Geometry: final body of the model. Coordinates: model frame, mm. A direction names the side the tool comes from. Coordinates: 2 decimals unless noted, no trailing zeros. Loops run counter-clockwise (first coordinate to the right, second up) from the corner with the lowest first, then second, coordinate; pieces in that order, holes last. Notation, with made-up numbers: (86.25, -34.5) - (140.25, -34.5) arc R20 ccw to (140.25, -16.5) - close; hole circle Ø5 at (74.5, 34). An arc over 180 degrees is marked (long way). Return JSON: item names as keys, results as strings.
Autodesk Inventor part; units mm, degrees
ref_plane "YZ Plane" through (0, 0, 0) normal (1, 0, 0) x (0, 1, 0)
ref_plane "XZ Plane" through (0, 0, 0) normal (0, 1, 0) x (-1, 0, 0)
ref_plane "XY Plane" through (0, 0, 0) normal (0, 0, 1) x (1, 0, 0)
sketch "Sketch1" plane through (0, 0, 0) normal (0, 1, 0) x (-1, 0, 0)
  line L0 (0, 0) -> (85.48, 0)
  line L1 (85.48, 0) -> (85.48, -127.76)
  line L2 (85.48, -127.76) -> (0, -127.76)
  line L3 (0, -127.76) -> (0, 0)
  line L4 (85.48, 0) -> (67.5195, -17.9605)
  line L5 (85.48, 0) -> (110.88, 0) construction
  line L6 (0, 0) -> (17.9605, -17.9605)
  line L7 (85.48, -127.76) -> (67.5195, -109.7995)
  line L8 (85.48, -127.76) -> (110.88, -127.76) construction
  line L9 (0, -127.76) -> (17.9605, -109.7995)
  line L10 (0, -127.76) -> (25.4, -127.76) construction
  dimension "d0" = 85.48
  dimension "d1" = 127.76
  dimension "d2" = 25.4
  dimension "d3" = 135
  dimension "d4" = 25.4
  dimension "d5" = 25.4
  dimension "d6" = 135
  dimension "d7" = 25.4
  dimension "d8" = 45
extrude "Extrusion1" add sketch "Sketch1" along normal blind 47.7
sketch "Sketch2" plane through (0, 0, 0) normal (0, -1, 0) x (1, 0, 0)
  line L0 (-85.48, 0) -> (0, 0)
  line L1 (0, 0) -> (-17.9605, -17.9605)
  line L2 (0, 0) -> (25.4, 0) construction
  line L3 (0, 0) -> (0, -127.76)
  line L4 (0, -127.76) -> (-17.9605, -109.7995)
  line L5 (0, -127.76) -> (25.4, -127.76) construction
  line L6 (-85.48, -127.76) -> (-85.48, 0)
  line L7 (-85.48, 0) -> (-67.5195, -17.9605)
  line L8 (-85.48, 0) -> (-60.08, 0) construction
  line L9 (0, -127.76) -> (-85.48, -127.76)
  line L10 (-85.48, -127.76) -> (-67.5195, -109.7995)
  line L11 (-85.48, -127.76) -> (-60.08, -127.76) construction
  dimension "d11" = 25.4
  dimension "d12" = 135
  dimension "d13" = 25.4
  dimension "d14" = 135
  dimension "d15" = 25.4
  dimension "d16" = 45
  dimension "d17" = 25.4
  dimension "d18" = 45
hole "Hole1" at (-17.9605, 0, -17.9605) at (-67.5195, 0, -17.9605) at (-67.5195, 0, -109.7995) at (-17.9605, 0, -109.7995) direction (0, 1, 0) diameter 3.683 depth 9.525 tip angle 118
sketch "Sketch4" plane through (0, 47.7, 0) normal (0, 1, 0) x (1, 0, 0)
  line L0 (0, -1.0521) -> (19.05, -1.0521) construction
  line L1 (0, 0) -> (0, 127.76)
  line L2 (0, 18.3507) -> (0, 0)
  line L3 (0, 0) -> (-18.7946, 0)
  line L4 (0, 0) -> (-14.1605, 0)
  line L5 (-14.1605, 0) -> (-14.1605, 16.256)
  line L6 (-14.1605, 16.256) -> (0, 16.256)
  line L7 (0, 16.256) -> (0, 0)
  dimension "d41" = 14.1605
  dimension "d42" = 16.256
hole "Hole2" at (-14.1605, 47.7, -16.256) direction (0, -1, 0) diameter 15 depth 35
pattern_linear "Rectangular Pattern1" count 4 spacing 19.05 along (-1, 0, 0) count 6 spacing 19.05 along (0, 0, -1) of "Hole2"
sketch "Sketch5" plane through (-85.48, 0, -127.76) normal (-1, 0, 0) x (0, 0, 1)
  line L0 (127.76, 0) -> (127.76, 47.7)
  line L1 (127.76, 0) -> (89.66, 0)
  line L2 (89.66, 0) -> (89.66, 6.35)
  line L3 (89.66, 6.35) -> (127.76, 6.35)
  line L4 (127.76, 6.35) -> (127.76, 0)
  line L5 (62.646, 6.35) -> (127.76, 6.35)
  line L6 (127.76, 6.35) -> (127.76, 0)
  line L7 (127.76, 0) -> (62.646, 0)
  line L8 (62.646, 0) -> (62.646, 6.35)
  dimension "d43" = 38.1
  dimension "d44" = 6.35
hole "Hole3" at (-85.48, 6.35, -38.1) direction (1, 0, 0) diameter 6.35 depth 31.75 tip angle 118
sketch "Sketch6" plane through (-85.48, 0, -127.76) normal (-1, 0, 0) x (0, 0, 1)
  line L0 (61.854, 6.5465) -> (127.76, 6.5465)
  line L1 (127.76, 6.5465) -> (127.76, 0.1965)
  line L2 (127.76, 0.1965) -> (61.854, 0.1965)
  line L3 (61.854, 0.1965) -> (61.854, 6.5465)
  point P0 (127.76, 0)
  dimension "d52" = 6.35
hole "Hole4" at (-85.48, 6.5465, -65.906) direction (1, 0, 0) diameter 3.175 depth 50.8 tip angle 118
sketch "Sketch7" plane through (0, 0, 0) normal (1, 0, 0) x (0, 0, -1)
  line L0 (127.76, 0) -> (0, 0)
  line L1 (127.76, 0) -> (89.66, 0)
  line L2 (89.66, 0) -> (89.66, 6.35)
  line L3 (89.66, 6.35) -> (127.76, 6.35)
  line L4 (127.76, 6.35) -> (127.76, 0)
  dimension "d60" = 38.1
  dimension "d61" = 6.35
hole "Hole5" at (0, 6.35, -89.66) direction (-1, 0, 0) diameter 6.35 depth 31.75 tip angle 118
properties part number "Thermal_topplate_4mL"
Item 1: Ray query, probe 1 along X at (y, z) = (25.5, -67); probe 2 along X at (y, z) = (33.5, -53.5); probe 3 along Y at (x, z) = (-53.5, -91). Return the intervals inside material, ascending. Write a range as from..to.
Worked out:
{"probe 1": "-85.48..-75.21, -67.41..-56.16, -48.36..-37.11, -29.31..-18.06, -10.26..0", "probe 2": "-85.48..-78.76, -63.86..-59.71, -44.81..-40.66, -25.76..-21.61, -6.71..0", "probe 3": "0..12.7"}
Item 2: First-contact query: pin 1 Ø4.5 at (x, z) = (-50, -38.5) entering from +Y. Flat tip, straight axial feed; report the tip coordinate or a pass-through.
Worked out:
{"pin 1": "y = 12.7"}
Item 3: Section query B-B, the plane y = 23. Count the separate pieces of the cut face and the enclosed holes in it, and give its area (3 significant figures).
Worked out:
{"separate pieces": "1", "enclosed holes": "24", "area": "6,680 mm^2"}
Item 4: Section query D-D, the plane z = -53.5. Return loops of the section in (x, y), and give its area (3 significant figures).
Worked out:
{"outline": "(-85.48, 0) - (0, 0) - (0, 47.7) - (-6.71, 47.7) - (-6.71, 12.7) - (-21.61, 12.7) - (-21.61, 47.7) - (-25.76, 47.7) - (-25.76, 12.7) - (-40.66, 12.7) - (-40.66, 47.7) - (-44.81, 47.7) - (-44.81, 12.7) - (-59.71, 12.7) - (-59.71, 47.7) - (-63.86, 47.7) - (-63.86, 12.7) - (-78.76, 12.7) - (-78.76, 47.7) - (-85.48, 47.7) - close", "area": "1,990 mm^2"}
Item 5: Reachability of faces 4 (the face through (-42, 24, 0)), 5 (the face through (-71, 12.7, -35)) from +Z, -Z, +X, -X, +Y, -Y: full face, straight path, thin tool, end or side. Return the list, or none.
Worked out:
{"face 4": "+Z, +X, -X, +Y, -Y", "face 5": "+Y"}
Item 6: Mould query, pull axis Y, two halves, no side actions, for faces 1 (the face through (-33.5, 30, -119)), 2 (the face through (-52, 12.7, -112)), 3 (the face through (-52.154, 6.374, -38.651)). Classes: +Y half, -Y half, draft (parallel to the pull), parting line (faces both ways), or undercut.
Worked out:
{"face 1": "draft", "face 2": "+Y half", "face 3": "undercut"}
